from build123d import *

# Parameters (mm, degrees)
SKETCH1_R                   = 20
BOSS_EXTRUDE1_DEPTH         = 1
SKETCH2_R                   = 13.25
CUT_EXTRUDE1_DEPTH          = 1
TAP_DRILL_FOR_M3X0_5_TAP1_D = 3.4


with BuildPart() as part:
    # Sketch1 → Boss-Extrude1 (new body)
    with BuildSketch(Plane.XY):
        Circle(SKETCH1_R)
    extrude(amount=BOSS_EXTRUDE1_DEPTH)

    # Sketch2 → Cut-Extrude1 (cut)
    with BuildSketch(Plane.XY.offset(1)):
        Circle(SKETCH2_R)
    extrude(amount=-CUT_EXTRUDE1_DEPTH, mode=Mode.SUBTRACT)

    # Tap Drill for M3x0.5 Tap1 (through all)
    with Locations(Plane.XY.offset(1)):
        with Locations((0, 17), (17, 0), (0, -17), (-17, 0)):
            Hole(TAP_DRILL_FOR_M3X0_5_TAP1_D / 2)


solid = part.part
Verification items for the finished model (mm, model axes). Coordinates: 2 decimals unless noted, no trailing zeros. Order: outer loops, then holes, each group sorted by start corner. A loop starts at its lowest first (then second) coordinate and runs counter-clockwise, first axis right, second up. Notation, with made-up numbers: M -7,-37.5 L 40,-37.5 A16 cw 40,-33.5 Z; hole C 71.25,40 d7. An arc over 180 degrees is marked long. One line per item, written item: value. Start each with the question number.
Item 1: Sectioned sample at C-C (x = -17). Enter the section's corners in (y, z).
Item 2: Mould release check, pull along X, two halves, no side actions. Record for faces 1 (the flat face through (4, -13, 0)), 2 (the cylindrical face through (15.38, 0.51, 0.49)), 3 (the cylindrical face through (-4.336, -19.524, 0.493)): released by +X, released by -X, zero draft, split by the parting line, or undercut.
Item 3: Sectioned sample at D-D (z = 0.8). Enter the section's corners in (x, y), then the cut area to 3 significant figures.
Item 4: Gauge pin test, flat end, axial feed: pin 1 (2 mm diameter, centred on x = 17, y = 0, fed in from +Z). Record the tip position at first contact, or that the pin passes through.
Item 5: Sectioned sample at A-A (y = 0). Enter the section's corners in (x, z), then the cut area to 3 significant figures.
Item 6: Scan lines: probe 1 along Y at (x, z) = (0, 0.75); probe 2 along X at (y, z) = (1.5, 0.4). Record each from-to range of solid material in increasing order.
Conclusion:
1. outline: M -10.54,0 L -1.7,0 L -1.7,1 L -10.54,1 Z; M 1.7,0 L 10.54,0 L 10.54,1 L 1.7,1 Z
2. face 1: zero draft
2. face 2: undercut
2. face 3: split by the parting line
3. outline: C 0,0 d40; hole C -17,0 d3.4; hole C 0,0 d26.5; hole C 0,-17 d3.4; hole C 0,17 d3.4; hole C 17,0 d3.4
3. area: 669 mm^2
4. pin 1: passes through
5. outline: M -20,0 L -18.7,0 L -18.7,1 L -20,1 Z; M -15.3,0 L -13.25,0 L -13.25,1 L -15.3,1 Z; M 13.25,0 L 15.3,0 L 15.3,1 L 13.25,1 Z; M 18.7,0 L 20,0 L 20,1 L 18.7,1 Z
5. area: 6.70 mm^2
6. probe 1: y = -20 to -18.7, -15.3 to -13.25, 13.25 to 15.3, 18.7 to 20
6. probe 2: x = -19.94 to -17.8, -16.2 to -13.16, 13.16 to 16.2, 17.8 to 19.94
